Could you check a few things on this model? Use its own coordinates, in mm. A direction names the side the tool comes from. Round coordinates to 2 decimals unless told otherwise and drop trailing zeros. Write each loop counter-clockwise with the first axis right and the second up, starting at its lowest first coordinate (ties: lowest second). Pieces come first, ordered by that corner, then holes. Notation, with made-up numbers: (-22, 2.25) - (3, 2.25) arc R25 ccw to (3, 28.25) - close; hole circle Ø1 at (-24.5, 52). An arc over 180 degrees is marked (long way). Put each result on its own line as item: value.
from build123d import *

# Parameters (mm, degrees)
BOSS_EXTRUDE1_DEPTH   = 11
BOSS_EXTRUDE1_2_DEPTH = 11
SKETCH1_R             = 2.5
BOSS_EXTRUDE1_3_DEPTH = 11
SKETCH1_11_R          = 2.5
BOSS_EXTRUDE2_DEPTH   = 1


with BuildPart() as part:
    # Sketch1 → Boss-Extrude1 (new, symmetric)
    with BuildSketch(Plane.XY):
        Polygon((0, -7), (0, -13), (1.8, -13), (1.8, -15.4), (3.6, -15.4), (6.1, -13), (6.1, -7), (3.6, -4.6), (1.8, -4.6), (1.8, -7), align=None)
    extrude(amount=BOSS_EXTRUDE1_DEPTH, both=True)



with BuildPart() as body_2:
    # Sketch1 → Boss-Extrude1 2 (new, symmetric)
    with BuildSketch(Plane.XY):
        Polygon((20, -7), (18.2, -7), (18.2, -4.6), (16.4, -4.6), (13.9, -7), (13.9, -13), (16.4, -15.4), (18.2, -15.4), (18.2, -13), (20, -13), align=None)
    extrude(amount=BOSS_EXTRUDE1_2_DEPTH, both=True)


with BuildPart() as body_3:
    # Sketch1 → Boss-Extrude1 3 (new, symmetric)
    with BuildSketch(Plane.XY):
        with Locations((10, -10)):
            Circle(SKETCH1_R)
    extrude(amount=BOSS_EXTRUDE1_3_DEPTH, both=True)


with BuildPart() as part_1:
    add(part.part)

    add(body_2.part)  # Boss-Extrude2 merges body 2

    add(body_3.part)  # Boss-Extrude2 merges body 3
    # Sketch1<11> → Boss-Extrude2 (add, symmetric)
    with BuildSketch(Plane.XY):
        Polygon((7, -1.8), (7, 0), (0, 0), (0, -7), (0.4, -7), (1.8, -7), (1.8, -4.6), (2.2, -4.6), (3.6, -4.6), (6.1, -7), (6.1, -13), (3.6, -15.4), (1.8, -15.4), (1.8, -13), (0.4, -13), (0, -13), (0, -20), (7, -20), (7, -18.2), (4.6, -18.2), (4.6, -16.4), (7, -13.9), (7.016, -13.9), (13, -13.9), (15.4, -16.4), (15.4, -18.2), (13, -18.2), (13, -19.6), (13, -20), (20, -20), (20, -13), (18.2, -13), (18.2, -15), (18.2, -15.4), (16.4, -15.4), (13.9, -13), (13.9, -12.6), (13.9, -7), (16.4, -4.6), (18.2, -4.6), (18.2, -7), (20, -7), (20, -6.6), (20, 0), (13, 0), (13, -1.8), (15.4, -1.8), (15.4, -3.6), (13, -6.1), (7, -6.1), (4.6, -3.6), (4.6, -1.8), align=None)
        with Locations((10, -10)):
            Circle(SKETCH1_11_R, mode=Mode.SUBTRACT)
    extrude(amount=BOSS_EXTRUDE2_DEPTH, both=True)


solid = part_1.part
(1) I'm going to push flat-ended pins straight in: pin 1 (0.7 mm diameter, centred on y = -6, z = -6, fed in from -X); pin 2 (1.4 mm diameter, centred on x = 3, z = 4.5, fed in from -Y); pin 3 (1 mm diameter, centred on y = -14, z = 8.5, fed in from +X); pin 4 (1.5 mm diameter, centred on y = -16.5, z = 5, fed in from +X). Where does each tip first touch, or does it pass through?
Values found:
pin 1: stops at x = 1.8
pin 2: stops at y = -15.4
pin 3: stops at x = 18.2
pin 4: passes through
(2) For faces 4 (the face through (14, -1.8, 0)), 5 (the face through (10, -6.1, 0)), 6 (the face through (3, -15.4, 6)), 7 (the face through (4.83, -14.22, 6.07)), 8 (the face through (3, -4.6, 6)), which set-ups out of +Z, -Z, +X, -X, +Y, -Y let a thin tool reach every point of the face, with its end or its side?
Values found:
face 4: +Z, -Z
face 5: +Z, -Z, +Y
face 6: +Z, +X, -X, -Y
face 7: +Z, -Y
face 8: +Z, +X, -X, +Y
(3) If we mould it in two halves opening along X, with no side actions, what happens to faces 1 (the face through (17, 0, 0)), 2 (the face through (20, -10, 0)), 3 (the face through (13, -19, 0))? For each: pulls with the +X half, pulls with the -X half, needs draft (parallel to the pull), parting line crosses it, or undercut.
Values found:
face 1: needs draft
face 2: pulls with the +X half
face 3: undercut
(4) Imagine slicing it at C-C, the plane x = 3.25. List the corners of the cut face in (y, z) for me, then the cut area to 3 significant figures.
Values found:
outline: (-20, -1) - (-15.4, -1) - (-15.4, -11) - (-4.6, -11) - (-4.6, -1) - (0, -1) - (0, 1) - (-4.6, 1) - (-4.6, 11) - (-15.4, 11) - (-15.4, 1) - (-20, 1) - close
area: 256 mm^2
(5) Imagine slicing it at B-B, the plane z = 7.25. List the corners of the cut face in (x, y) for me, then the cut area to 3 significant figures.
Values found:
outline: (0, -13) - (1.8, -13) - (1.8, -15.4) - (3.6, -15.4) - (6.1, -13) - (6.1, -7) - (3.6, -4.6) - (1.8, -4.6) - (1.8, -7) - (0, -7) - close; circle Ø5 at (10, -10); (13.9, -13) - (16.4, -15.4) - (18.2, -15.4) - (18.2, -13) - (20, -13) - (20, -7) - (18.2, -7) - (18.2, -4.6) - (16.4, -4.6) - (13.9, -7) - close
area: 122 mm^2
(6) Imagine slicing it at D-D, the plane z = -0.25. List the corners of the cut face in (x, y) for me.
Values found:
outline: (0, -20) - (7, -20) - (7, -18.2) - (4.6, -18.2) - (4.6, -16.4) - (7, -13.9) - (13, -13.9) - (15.4, -16.4) - (15.4, -18.2) - (13, -18.2) - (13, -20) - (20, -20) - (20, 0) - (13, 0) - (13, -1.8) - (15.4, -1.8) - (15.4, -3.6) - (13, -6.1) - (7, -6.1) - (4.6, -3.6) - (4.6, -1.8) - (7, -1.8) - (7, 0) - (0, 0) - close
(7) Imagine slicing it at A-A, the plane y = -17. List the corners of the cut face in (x, z) for me.
Values found:
outline: (0, -1) - (4.6, -1) - (4.6, 1) - (0, 1) - close; (15.4, -1) - (20, -1) - (20, 1) - (15.4, 1) - close
(8) Please list where these lines run through material, in increasing order: probe 1 along X at (y, z) = (-10.5, -9.5); probe 2 along Y at (x, z) = (1.5, -1.5); probe 3 along X at (y, z) = (-6.75, 4.5). Write a range as from..to.
Values found:
probe 1: x = 0..6.1, 7.55..12.45, 13.9..20
probe 2: y = -13..-7
probe 3: x = 1.8..5.84, 14.16..18.2
